```python
from build123d import *

# Parameters (mm, degrees)
F1_DEPTH = 280
F3_DEPTH = 280


with BuildPart() as f1:
    # F0 (on Front) → F1 (new body)
    with BuildSketch(Plane.XZ):
        with BuildLine():
            Line((-26.003272, 3.696673), (-26.246255, 18.303327))
            ThreePointArc((-26.246255, 18.303327), (-26.305987, 18.442593), (-26.446228, 18.5))
            Line((-26.446228, 18.5), (-27.552839, 18.5))
            ThreePointArc((-27.552839, 18.5), (-27.693074, 18.442597), (-27.752811, 18.303339))
            Line((-27.752811, 18.303339), (-27.996716, 3.696661))
            Line((-27.996716, 3.696661), (-27.996716, -9.5))
            Line((-27.996716, -9.5), (-21.35, -9.5))
            ThreePointArc((-21.35, -9.5), (-21.208579, -9.441421), (-21.15, -9.3))
            Line((-21.15, -9.3), (-21.15, -3.7))
            ThreePointArc((-21.15, -3.7), (-21.091421, -3.558579), (-20.95, -3.5))
            Line((-20.95, -3.5), (0, -3.502103))
            Line((0, -3.502103), (0, -1.502103))
            Line((0, -1.502103), (-4.654982, -1.502103))
            ThreePointArc((-4.654982, -1.502103), (-4.796403, -1.443525), (-4.854982, -1.302103))
            Line((-4.854982, -1.302103), (-4.854982, 1.297897))
            ThreePointArc((-4.854982, 1.297897), (-4.796403, 1.439318), (-4.654982, 1.497897))
            Line((-4.654982, 1.497897), (0, 1.497897))
            Line((0, 1.497897), (0, 18.497629))
            Line((0, 18.497629), (-0.55284, 18.497629))
            ThreePointArc((-0.55284, 18.497629), (-0.693076, 18.440226), (-0.752812, 18.300968))
            Line((-0.752812, 18.300968), (-0.996713, 3.694558))
            ThreePointArc((-0.996713, 3.694558), (-1.056449, 3.5553), (-1.196685, 3.497897))
            Line((-1.196685, 3.497897), (-5.550001, 3.497897))
            ThreePointArc((-5.550001, 3.497897), (-5.691423, 3.556475), (-5.750001, 3.697897))
            Line((-5.750001, 3.697897), (-5.750001, 18.3))
            ThreePointArc((-5.750001, 18.3), (-5.80858, 18.441421), (-5.950001, 18.5))
            Line((-5.950001, 18.5), (-7.302839, 18.5))
            ThreePointArc((-7.302839, 18.5), (-7.443074, 18.442597), (-7.502811, 18.303339))
            Line((-7.502811, 18.303339), (-7.746716, 3.696661))
            ThreePointArc((-7.746716, 3.696661), (-7.806452, 3.557403), (-7.946688, 3.5))
            Line((-7.946688, 3.5), (-12.303299, 3.5))
            ThreePointArc((-12.303299, 3.5), (-12.44354, 3.557407), (-12.503272, 3.696673))
            Line((-12.503272, 3.696673), (-12.746255, 18.303327))
            ThreePointArc((-12.746255, 18.303327), (-12.805987, 18.442593), (-12.946228, 18.5))
            Line((-12.946228, 18.5), (-14.052839, 18.5))
            ThreePointArc((-14.052839, 18.5), (-14.193074, 18.442597), (-14.252811, 18.303339))
            Line((-14.252811, 18.303339), (-14.496716, 3.696661))
            ThreePointArc((-14.496716, 3.696661), (-14.556452, 3.557403), (-14.696688, 3.5))
            Line((-14.696688, 3.5), (-19.053299, 3.5))
            ThreePointArc((-19.053299, 3.5), (-19.19354, 3.557407), (-19.253272, 3.696673))
            Line((-19.253272, 3.696673), (-19.496255, 18.303327))
            ThreePointArc((-19.496255, 18.303327), (-19.555987, 18.442593), (-19.696228, 18.5))
            Line((-19.696228, 18.5), (-20.802839, 18.5))
            ThreePointArc((-20.802839, 18.5), (-20.943074, 18.442597), (-21.002811, 18.303339))
            Line((-21.002811, 18.303339), (-21.246716, 3.696661))
            ThreePointArc((-21.246716, 3.696661), (-21.306452, 3.557403), (-21.446688, 3.5))
            Line((-21.446688, 3.5), (-25.803299, 3.5))
            ThreePointArc((-25.803299, 3.5), (-25.94354, 3.557407), (-26.003272, 3.696673))
        make_face()
    extrude(amount=F1_DEPTH)

    # F2 (on face) → F3 (join)
    with BuildSketch(Plane.XZ.offset(280)):
        with BuildLine():
            Line((-27.996716, -9.5), (-27.996716, -7.503925))
            Line((-27.996716, -7.503925), (-32.788628, -7.503925))
            ThreePointArc((-32.788628, -7.503925), (-32.865164, -7.488701), (-32.930049, -7.445347))
            Line((-32.930049, -7.445347), (-38.24641, -2.128986))
            ThreePointArc((-38.24641, -2.128986), (-38.387831, -2.070407), (-38.529253, -2.128986))
            Line((-38.529253, -2.128986), (-39.30707, -2.906803))
            ThreePointArc((-39.30707, -2.906803), (-39.365649, -3.048225), (-39.30707, -3.189646))
            Line((-39.30707, -3.189646), (-33.055295, -9.441421))
            ThreePointArc((-33.055295, -9.441421), (-32.99041, -9.484776), (-32.913873, -9.5))
            Line((-32.913873, -9.5), (-27.996716, -9.5))
        make_face()
        with BuildLine():
            ThreePointArc((-32.788628, -2.003925), (-32.865164, -1.988701), (-32.930049, -1.945347))
            Line((-32.930049, -1.945347), (-38.24641, 3.371014))
            ThreePointArc((-38.24641, 3.371014), (-38.387831, 3.429593), (-38.529253, 3.371014))
            Line((-38.529253, 3.371014), (-39.30707, 2.593197))
            ThreePointArc((-39.30707, 2.593197), (-39.365649, 2.451775), (-39.30707, 2.310354))
            Line((-39.30707, 2.310354), (-33.055295, -3.941421))
            ThreePointArc((-33.055295, -3.941421), (-32.99041, -3.984776), (-32.913873, -4))
            Line((-32.913873, -4), (-27.996716, -4))
            Line((-27.996716, -4), (-27.996716, -2.003925))
            Line((-27.996716, -2.003925), (-32.788628, -2.003925))
        make_face()
        with BuildLine():
            ThreePointArc((-32.788628, 3.496075), (-32.865164, 3.511299), (-32.930049, 3.554653))
            Line((-32.930049, 3.554653), (-38.24641, 8.871014))
            ThreePointArc((-38.24641, 8.871014), (-38.387831, 8.929593), (-38.529253, 8.871014))
            Line((-38.529253, 8.871014), (-39.30707, 8.093197))
            ThreePointArc((-39.30707, 8.093197), (-39.365649, 7.951775), (-39.30707, 7.810354))
            Line((-39.30707, 7.810354), (-33.055295, 1.558579))
            ThreePointArc((-33.055295, 1.558579), (-32.99041, 1.515224), (-32.913873, 1.5))
            Line((-32.913873, 1.5), (-27.996716, 1.5))
            Line((-27.996716, 1.5), (-27.996716, 3.496075))
            Line((-27.996716, 3.496075), (-32.788628, 3.496075))
        make_face()
    extrude(amount=-F3_DEPTH)

    # F4: F1 across face


with BuildPart() as f1_1:
    add(f1.part)
    add(f1.part.mirror(Plane(origin=(0, -140, 9.997763), x_dir=(0, 1, 0), z_dir=(1, 0, 0))))


solid = f1_1.part
```
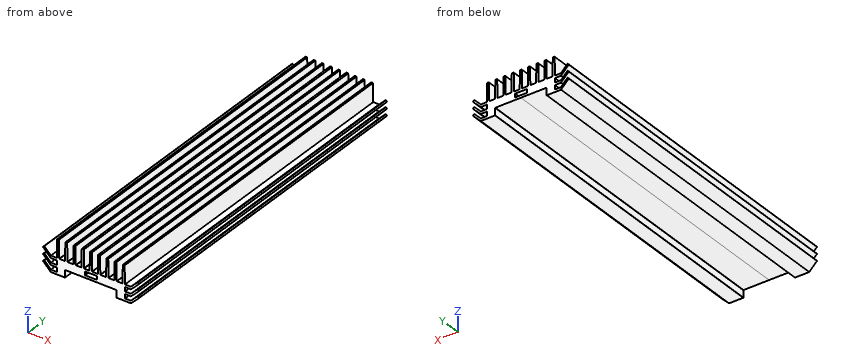
Geometry: final body of the model. Coordinates: model frame, mm. Round coordinates to 2 decimals unless told otherwise and drop trailing zeros. Write each question's results on one line, items separated by ' | '.
Item 1: Line query: probe 1 along X at (y, z) = (-229.5, -5.5); probe 2 along X at (y, z) = (-30, -5); probe 3 along Z at (x, y) = (2, -133.5). Output: solid intervals per line, ascending. Write a range as [from, to].
Answers below:
probe 1: x = [-37, -34.88], [-28, -21.15], [21.15, 28], [34.88, 37] | probe 2: x = [-37.5, -35.38], [-28, -21.15], [21.15, 28], [35.38, 37.5] | probe 3: z = [-3.5, -1.5], [1.5, 3.5]
Item 2: Pin query (flat end, axial travel): pin 1 Ø2.5 at (x, y) = (-30.5, -197.5) entering from +Z; pin 2 Ø2 at (y, z) = (-51.5, 11) entering from +X; pin 3 Ø4 at (y, z) = (-81, 0) entering from -X. Return the tip coordinate at first contact, or that it passes through.
Answers below:
pin 1: stops at z = 3.5 | pin 2: stops at x = 27.89 | pin 3: stops at x = -39
Item 3: Cut plane A-A on z = 15. State how many separate pieces and enclosed holes the cut face has, and give its area (3 significant figures).
Answers below:
separate pieces: 9 | enclosed holes: 0 | area: 4,180 mm²
